Verification items for the finished model (mm, model axes). Face numbers are marked on the shaded views. Coordinates: 2 decimals unless noted, no trailing zeros. Loops run counter-clockwise (first coordinate to the right, second up) from the corner with the lowest first, then second, coordinate; pieces in that order, holes last. Notation, with made-up numbers: (87, 88.5) -> (134, 88.5) arc R14 ccw to (134, 99.5) -> close; hole circle Ø9 at (51, -35). An arc over 180 degrees is marked (long way). Write item = value, one per line.
Autodesk Inventor part; units mm, degrees
ref_plane "YZ Plane" through (0, 0, 0) normal (1, 0, 0) x (0, 1, 0)
ref_plane "XZ Plane" through (0, 0, 0) normal (0, 1, 0) x (-1, 0, 0)
ref_plane "XY Plane" through (0, 0, 0) normal (0, 0, 1) x (1, 0, 0)
sketch "スケッチ1" plane through (0, 0, 0) normal (1, 0, 0) x (0, 1, 0)
  circle A0 centre (0, 0) radius 4.6
  line L0 (4.6, 0) -> (2.3, 3.9837)
  line L1 (2.3, 3.9837) -> (-2.3, 3.9837)
  line L2 (-2.3, 3.9837) -> (-4.6, 0)
  line L3 (-4.6, 0) -> (-2.3, -3.9837)
  line L4 (2.3, -3.9837) -> (-2.3, -3.9837)
  line L5 (2.3, -3.9837) -> (4.6, 0)
  circle A1 centre (0, 0) radius 2.5
  point P0 (-2.3, -3.9837)
  dimension "d0" = 9.2
  dimension "d3" = 360
  dimension "d5" = 5
extrude "押し出し1" add sketch "スケッチ1" along normal blind 4 contours L5 L4 L3 L2 L1 L0
properties part number "5min-nut" material "アルミニウム 6061"
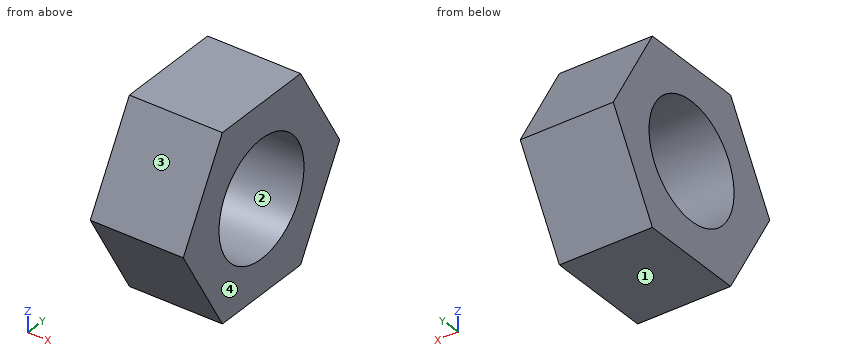
1) Sectioned sample at B-B, the plane x = 3.25. Record the cut outline in (y, z).
Ans:
outline = (-4.6, 0) -> (-2.3, -3.98) -> (2.3, -3.98) -> (4.6, 0) -> (2.3, 3.98) -> (-2.3, 3.98) -> close; hole circle Ø5 at (0, 0)
2) Sectioned sample at D-D, the plane y = -3.25. Record the cut outline in (x, z), plus the area to 3 significant figures.
Ans:
outline = (0, -2.34) -> (4, -2.34) -> (4, 2.34) -> (0, 2.34) -> close
area = 18.7 mm2
3) Depth check by flat-ended pin: pin 1 Ø2 at (x, z) = (3.5, -1.5) entering from +Y; pin 2 Ø2 at (x, z) = (2, -2) entering from +Y. Enter the tip coordinate at first touch or a pass-through.
Ans:
pin_1 = 4.31
pin_2 = 4.02
4) Sectioned sample at A-A, the plane y = 1.5. Record the cut outline in (x, z).
Ans:
outline = (0, -3.98) -> (4, -3.98) -> (4, -2) -> (0, -2) -> close; (0, 2) -> (4, 2) -> (4, 3.98) -> (0, 3.98) -> close
5) Sectioned sample at C-C, the plane z = -1. Record the cut outline in (x, y).
Ans:
outline = (0, -4.02) -> (4, -4.02) -> (4, -2.29) -> (0, -2.29) -> close; (0, 2.29) -> (4, 2.29) -> (4, 4.02) -> (0, 4.02) -> close
6) Release check for a two-part mould opening along Z. For the marked faces 1, 2, 3 and 4 record: pulls with the +Z half, pulls with the -Z half, needs draft (parallel to the pull), parting line crosses it, or undercut.
Ans:
face_1 = pulls with the -Z half
face_2 = undercut
face_3 = pulls with the +Z half
face_4 = needs draft
7) Material ranges on line 1 (Z direction, x = 1.15, y = 0); line 2 (Y direction, x = 3, z = 2.25); line 3 (Z direction, x = 0.3, y = -0.75), recorded low to high.
Ans:
line_1 = -3.98 to -2.5, 2.5 to 3.98
line_2 = -3.3 to -1.09, 1.09 to 3.3
line_3 = -3.98 to -2.38, 2.38 to 3.98
